Answer from the drawing. Dimensions are ordinates in mm from the lowest x, y and z of the part. Coordinates: 2 decimals unless noted, no trailing zeros. Order: outer loops, then holes, each group sorted by start corner. A loop starts at its lowest first (then second) coordinate and runs counter-clockwise, first axis right, second up.
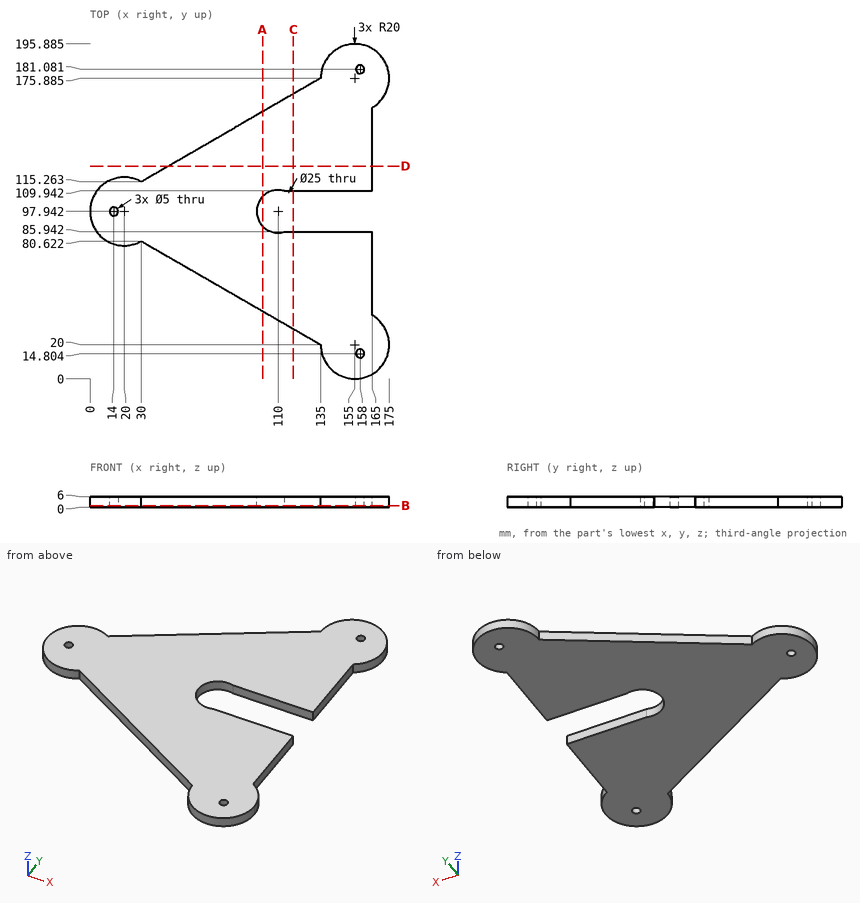
1. The part is cut by section D-D (y = 124.5). Determine the outline of the cut face in (x, z), plus the area to 3 significant figures.
2. The part is cut by section A-A (x = 101). Determine the outline of the cut face in (y, z) (1 decimal).
3. Flat-ended cylindrical pins translate along their axes: pin 1 (3 mm diameter, centred on x = 79, z = 4, fed in from -Y) (1 decimal); pin 2 (1 mm diameter, centred on x = 57, z = 5, fed in from +Y); pin 3 (1.5 mm diameter, centred on x = 54, z = 1, fed in from -Y). Find the tip coordinate at first contact, or state that the pin passes through.
4. The part is cut by section C-C (x = 119). Determine the outline of the cut face in (y, z).
5. Consider probe 1 along Y at (x, z) = (158, 3.7); probe 2 along Y at (x, z) = (30, 4.3); probe 3 along Y at (x, z) = (14, 2.7). Determine where each line is inside the solid, lowest interval first.
6. The part is cut by section B-B (z = 0.9). Count the separate pieces of the cut face and the enclosed holes in it, plus the area to 3 significant figures.
Worked out:
1. outline: (46, 0) - (165, 0) - (165, 6) - (46, 6) - close
1. area: 714 mm2
2. outline: (39.6, 0) - (89.3, 0) - (89.3, 6) - (39.6, 6) - close; (106.6, 0) - (156.3, 0) - (156.3, 6) - (106.6, 6) - close
3. pin 1: stops at y = 51.5
3. pin 2: stops at y = 131.14
3. pin 3: stops at y = 66.33
4. outline: (29.24, 0) - (85.94, 0) - (85.94, 6) - (29.24, 6) - close; (109.94, 0) - (166.65, 0) - (166.65, 6) - (109.94, 6) - close
5. probe 1: y = 0.23 to 12.3, 17.3 to 85.94, 109.94 to 178.58, 183.58 to 195.66
5. probe 2: y = 80.62 to 115.26
5. probe 3: y = 78.86 to 95.44, 100.44 to 117.02
6. separate pieces: 1
6. enclosed holes: 3
6. area: 15,600 mm2
